from build123d import *

# Parameters (mm, degrees)
EXTRUDE_1_DEPTH              = 30
HOLE_WIZARD_M3_1_D           = 3.2
HOLE_WIZARD_M3_1_CBORE_D     = 6.5
HOLE_WIZARD_M3_1_CBORE_DEPTH = 3
FILLET_1_R                   = 15
CUT_EXTRUDE_1782_DEPTH       = 90.635744244
FILLET_2_R                   = 5
EXTRUDE_2_DEPTH              = 11
FILLET_3_R                   = 8


with BuildPart() as part:
    # ｽｹｯﾁ1 → ﾎﾞｽ - 押し出し1 (new body)
    with BuildSketch(Plane.XY):
        with BuildLine():
            Line((8, 59.464274989), (8, 28))
            Line((8, 28), (-22, 28))
            Line((-22, 28), (-22, 29))
            Line((-22, 29), (-28, 29))
            Line((-28, 29), (-28, -29))
            Line((-28, -29), (-22, -29))
            Line((-22, -29), (-22, -28))
            Line((-22, -28), (8, -28))
            Line((8, -28), (8, -59.464274989))
            ThreePointArc((8, -59.464274989), (-60, 0), (8, 59.464274989))
        make_face()
    extrude(amount=EXTRUDE_1_DEPTH)

    # M3 穴付きねじ用座ぐり穴1 (through all)
    with Locations(Plane(origin=(0, 45, 30), x_dir=(1, 0, 0), z_dir=(0, 0, 1))):
        with Locations((0, 0), (-45, -45), (0, -90)):
            CounterBoreHole(HOLE_WIZARD_M3_1_D / 2, HOLE_WIZARD_M3_1_CBORE_D / 2, HOLE_WIZARD_M3_1_CBORE_DEPTH)

    # ﾌｨﾚｯﾄ1
    fillet_1_edges = [part.edges().sort_by_distance(p)[0] for p in [
        (8, 59.464274989, 15),
        (8, -59.464274989, 15),
    ]]
    fillet(fillet_1_edges, radius=FILLET_1_R)

    # ｽｹｯﾁ3 → Cut-Extrude 1782 (cut, through all)
    with BuildSketch(Plane.XY):
        with BuildLine():
            Line((-28, 29), (-28, 20.55))
            ThreePointArc((-28, 20.55), (-32.225, 24.775), (-28, 29))
        make_face()
        with BuildLine():
            Line((-28, -29), (-28, -20.55))
            ThreePointArc((-28, -20.55), (-32.225, -24.775), (-28, -29))
        make_face()
    extrude(amount=CUT_EXTRUDE_1782_DEPTH, mode=Mode.SUBTRACT)

    # ﾌｨﾚｯﾄ2
    fillet_2_edges = [part.edges().sort_by_distance(p)[0] for p in [
        (8, 28, 15),
        (8, -28, 15),
        (-28, 20.55, 15),
        (-28, -20.55, 15),
    ]]
    fillet(fillet_2_edges, radius=FILLET_2_R)

    # ｽｹｯﾁ4 → ﾎﾞｽ - 押し出し2 (add)
    with BuildSketch(Plane.XY.offset(30)):
        with BuildLine():
            Line((8, 44.452221542), (8, 61.887817316))
            ThreePointArc((8, 61.887817316), (-0.707298954, 66.574651642), (-10.577777778, 67.172245885))
            ThreePointArc((-10.577777778, 67.172245885), (-68, 0), (-10.577777778, -67.172245885))
            ThreePointArc((-10.577777778, -67.172245885), (-0.707298954, -66.574651642), (8, -61.887817316))
            Line((8, -61.887817316), (8, -44.452221542))
            ThreePointArc((8, -44.452221542), (2.746794345, -55.853975793), (-9.333333333, -59.269628722))
            ThreePointArc((-9.333333333, -59.269628722), (-60, 0), (-9.333333333, 59.269628722))
            ThreePointArc((-9.333333333, 59.269628722), (2.746794345, 55.853975793), (8, 44.452221542))
        make_face()
    extrude(amount=-EXTRUDE_2_DEPTH)

    # ﾌｨﾚｯﾄ3
    fillet_3_edges = [part.edges().sort_by_distance(p)[0] for p in [
        (8, -61.887817316, 24.5),
        (8, 61.887817316, 24.5),
    ]]
    fillet(fillet_3_edges, radius=FILLET_3_R)


solid = part.part
Design review of the part built by this model. Coordinates are the model's own, in mm. A direction names the side the tool comes from. Give positions to 0.01 mm unless a question says otherwise; leave off trailing zeros. Loops run counter-clockwise (first coordinate to the right, second up) from the corner with the lowest first, then second, coordinate; pieces in that order, holes last. Notation, with made-up numbers: (55.5, -35) -> (113.5, -35) arc R25 cw to (113.5, -12) -> close; hole circle Ø5 at (64.25, 9.5). An arc over 180 degrees is marked (long way). One line per question, with ' | ' between items. Start each with the question number.
(1) We need section D-D (x = 0). State the section outline as (y, z) points, and give its area (3 significant figures).
(2) Draft analysis for pull direction X (two halves, no side actions). For faces 5 (the face through (-28.6, -19.4, 15.2)), 6 (the face through (-25, 29, 15)), 7 (the face through (-3.128, 67.124, 24.577)), state which applies: +X half, -X half, draft (parallel to the pull), parting line (faces both ways), or undercut.
(3) For faces 1 (the face through (-67.987, 1.347, 24.577)), 2 (the face through (-25, -29, 15)), 3 (the face through (-9, 28, 15)), 4 (the face through (-0.705, -48.173, 28.521)), list the 3-axis set-ups (+Z, -Z, +X, -X, +Y, -Y) from which the entire face can be reached by the end or side of a thin tool; tool diameter is ignored.
(4) For line 1 (Y direction, x = 0, z = 12.25); line 2 (Y direction, x = -30, z = 8.75); line 3 (Y direction, x = 0, z = 21.5), list the stretches that pass through material, from the lowest coordinate up.
(5) We need section C-C (z = 24.5). State the section outline as (x, y) points (3 decimals).
(6) We need section A-A (y = 0). State the section outline as (x, z) points.
(7) Insertion check: P1, Ø5, axis at x = -24.5, z = 21, coming from the -Y side; P2, Ø3, axis at x = -1, y = 44.5, coming from the +Z side; P3, Ø6, axis at x = 0.5, z = 21.5, coming from the +Y side. Each pin has a flat end and moves straight along its axis. Give the tip position at first contact, or say it passes through.
(8) We need section B-B (x = -15). State the section outline as (y, z) points.
The answers:
1) outline: (-66.36, 19) -> (-57.72, 19) -> (-57.72, 0) -> (-46.6, 0) -> (-46.6, 27) -> (-48.25, 27) -> (-48.25, 30) -> (-66.36, 30) -> close; (-43.4, 0) -> (-28, 0) -> (-28, 30) -> (-41.75, 30) -> (-41.75, 27) -> (-43.4, 27) -> close; (28, 0) -> (43.4, 0) -> (43.4, 27) -> (41.75, 27) -> (41.75, 30) -> (28, 30) -> close; (46.6, 0) -> (57.72, 0) -> (57.72, 19) -> (66.36, 19) -> (66.36, 30) -> (48.25, 30) -> (48.25, 27) -> (46.6, 27) -> close | area: 1,760 mm^2
2) face 5: +X half | face 6: undercut | face 7: parting line
3) face 1: +Z, -Z, -X | face 2: +Z, -Z | face 3: +Z, -Z, +X | face 4: +Z
4) line 1: y = -57.72 to -46.6, -43.4 to -28, 28 to 43.4, 46.6 to 57.72 | line 2: y = -51.96 to -28.5, -21.02 to 21.02, 28.5 to 51.96 | line 3: y = -66.36 to -46.6, -43.4 to -28, 28 to 43.4, 46.6 to 66.36
5) outline: (-30.29, -21.224) arc R5 ccw to (-28, -17.023) -> (-28, 17.023) arc R5 ccw to (-30.29, 21.224) arc R4.225 cw to (-28, 29) -> (-22, 29) -> (-22, 28) -> (3, 28) arc R5 ccw to (8, 33) -> (8, 57.719) arc R8 ccw to (3.733, 64.794) arc R23 ccw to (-10.578, 67.172) arc R68 ccw to (-10.578, -67.172) arc R23 ccw to (3.733, -64.794) arc R8 ccw to (8, -57.719) -> (8, -33) arc R5 ccw to (3, -28) -> (-22, -28) -> (-22, -29) -> (-28, -29) arc R4.225 cw to start; hole circle Ø3.2 at (-45, 0); hole circle Ø3.2 at (0, -45); hole circle Ø3.2 at (0, 45)
6) outline: (-68, 19) -> (-60, 19) -> (-60, 0) -> (-46.6, 0) -> (-46.6, 27) -> (-48.25, 27) -> (-48.25, 30) -> (-68, 30) -> close; (-43.4, 0) -> (-28, 0) -> (-28, 30) -> (-41.75, 30) -> (-41.75, 27) -> (-43.4, 27) -> close
7) P1: stops at y = -64.34 | P2: stops at z = 27 | P3: stops at y = 67.01
8) outline: (-66.32, 19) -> (-58.09, 19) -> (-58.09, 0) -> (-28, 0) -> (-28, 30) -> (-66.32, 30) -> close; (28, 0) -> (58.09, 0) -> (58.09, 19) -> (66.32, 19) -> (66.32, 30) -> (28, 30) -> close
